from build123d import *

# Parameters (mm, degrees)
BOSS_EXTRUDE1_DEPTH   = 4
BOSS_EXTRUDE1_2_DEPTH = 4
BOSS_EXTRUDE3_DEPTH   = 4
FILLET2_R             = 1
SKETCH4_W             = 14.347682942
SKETCH4_H             = 12.983957321
BOSS_EXTRUDE4_DEPTH   = 15
SKETCH6_W             = 14.347682942
SKETCH6_H             = 3
BOSS_EXTRUDE6_DEPTH   = 10
CUT_EXTRUDE1_REACH    = 49.733
SKETCH7_R             = 1.5
CAVITY2_START         = 21.87499999
CAVITY2_DEPTH         = 1.12500001
SKETCH8_W             = 3
SKETCH8_H             = 13
BOSS_EXTRUDE7_DEPTH   = 10
CUT_EXTRUDE2_REACH    = 71.123
SKETCH10_R            = 1.5


# Read off the part's stored shape, not the designer's step: Cavity2
with BuildPart() as part:
    # Sketch1 → Boss-Extrude1 (new body)
    with BuildSketch(Plane(origin=(0, 0, 0), x_dir=(1, 0, 0), z_dir=(0, 1, 0))):
        with BuildLine():
            Line((-23.6, 10.542278437), (-17, 10.542278437))
            ThreePointArc((-17, 10.542278437), (-15.475, 9.017278437), (-17, 7.492278437))
            Line((-17, 7.492278437), (-23.6, 7.492278437))
            ThreePointArc((-23.6, 7.492278437), (-25.125, 9.017278437), (-23.6, 10.542278437))
        make_face()
    extrude(amount=BOSS_EXTRUDE1_DEPTH)



with BuildPart() as body_2:
    # Sketch1 → Boss-Extrude1 2 (new body)
    with BuildSketch(Plane(origin=(0, 0, 0), x_dir=(1, 0, 0), z_dir=(0, 1, 0))):
        with BuildLine():
            Line((23.6, 7.492278437), (17, 7.492278437))
            ThreePointArc((17, 7.492278437), (15.475, 9.017278437), (17, 10.542278437))
            Line((17, 10.542278437), (23.6, 10.542278437))
            ThreePointArc((23.6, 10.542278437), (25.125, 9.017278437), (23.6, 7.492278437))
        make_face()
    extrude(amount=BOSS_EXTRUDE1_2_DEPTH)


with BuildPart() as part_1:
    add(part.part)

    add(body_2.part)  # Boss-Extrude3 merges body 2
    # Sketch3 → Boss-Extrude3 (add)
    with BuildSketch(Plane(origin=(0, 4, 0), x_dir=(1, 0, 0), z_dir=(0, 1, 0))):
        with BuildLine():
            ThreePointArc((15.475, 9.017278437), (15.921662159, 7.938940596), (17, 7.492278437))
            Line((17, 7.492278437), (23.6, 7.492278437))
            ThreePointArc((23.6, 7.492278437), (24.678337841, 7.938940596), (25.125, 9.017278437))
            Line((25.125, 9.017278437), (25.125, 17.305889592))
            Line((25.125, 17.305889592), (25.125, 34.117278437))
            Line((25.125, 34.117278437), (-25.125, 34.117278437))
            Line((-25.125, 34.117278437), (-25.125, 17.305889592))
            Line((-25.125, 17.305889592), (-25.125, 9.017278437))
            ThreePointArc((-25.125, 9.017278437), (-24.678337841, 10.095616278), (-23.6, 10.542278437))
            Line((-23.6, 10.542278437), (-17, 10.542278437))
            ThreePointArc((-17, 10.542278437), (-15.921662159, 10.095616278), (-15.475, 9.017278437))
            Line((-15.475, 9.017278437), (-15.475, 14.117278437))
            Line((-15.475, 14.117278437), (15.475, 14.117278437))
            Line((15.475, 14.117278437), (15.475, 9.017278437))
        make_face()
        with BuildLine():
            Line((-17, 10.542278437), (-23.6, 10.542278437))
            ThreePointArc((-23.6, 10.542278437), (-25.125, 9.017278437), (-23.6, 7.492278437))
            Line((-23.6, 7.492278437), (-17, 7.492278437))
            ThreePointArc((-17, 7.492278437), (-15.475, 9.017278437), (-17, 10.542278437))
        make_face()
    extrude(amount=BOSS_EXTRUDE3_DEPTH)

    # Fillet2
    fillet2_edges = [part_1.edges().sort_by_distance(p)[0] for p in [
        (-25.125, 8, -21.567278437),
        (15.475, 8, -11.567278437),
        (-24.678337841, 8, -7.938940596),
        (-20.3, 8, -7.492278437),
        (-15.921662159, 8, -7.938940596),
        (-15.475, 8, -11.567278437),
        (15.921662159, 8, -7.938940596),
        (20.3, 8, -7.492278437),
        (24.678337841, 8, -7.938940596),
        (25.125, 8, -21.567278437),
    ]]
    fillet(fillet2_edges, radius=FILLET2_R)

    # Sketch4 → Boss-Extrude4 (add)
    with BuildSketch(Plane(origin=(0, 8, 0), x_dir=(1, 0, 0), z_dir=(0, 1, 0))):
        with Locations((-7.885296824, 27.625299777)):
            Rectangle(SKETCH4_W, SKETCH4_H)
    extrude(amount=BOSS_EXTRUDE4_DEPTH)

    # Sketch6 → Boss-Extrude6 (add)
    with BuildSketch(Plane(origin=(0, 23, 0), x_dir=(1, 0, 0), z_dir=(0, 1, 0))):
        with Locations((-7.885296824, 32.617278437)):
            Rectangle(SKETCH6_W, SKETCH6_H)
    extrude(amount=BOSS_EXTRUDE6_DEPTH)

    # Sketch7 → Cut-Extrude1 (cut, up to next)
    with BuildSketch(Plane.XY.offset(-31.117278437), mode=Mode.PRIVATE) as cut_extrude1_sk1:
        with Locations((-11.819138295, 28.245)):
            Circle(SKETCH7_R)
    cut_extrude1_tool1 = extrude(cut_extrude1_sk1.sketch, amount=-CUT_EXTRUDE1_REACH, mode=Mode.PRIVATE) & part_1.part
    # Sketch7 → Cut-Extrude1 (cut, up to next)
    with BuildSketch(Plane.XY.offset(-31.117278437), mode=Mode.PRIVATE) as cut_extrude1_sk2:
        with Locations((-5.789138295, 28.245)):
            Circle(SKETCH7_R)
    cut_extrude1_tool2 = extrude(cut_extrude1_sk2.sketch, amount=-CUT_EXTRUDE1_REACH, mode=Mode.PRIVATE) & part_1.part
    add(cut_extrude1_tool1.solids().sort_by_distance((-11.819138, 28.245, -31.117278))[0], mode=Mode.SUBTRACT)
    add(cut_extrude1_tool2.solids().sort_by_distance((-5.789138, 28.245, -31.117278))[0], mode=Mode.SUBTRACT)

    # Cavity2 outline → Cavity2 (cut)
    with BuildSketch(Plane(origin=(0, 0, 0), x_dir=(1, 0, 0), z_dir=(0, 1, 0)).offset(CAVITY2_START)):
        Polygon((-0.711455353, 21.133321116), (-0.711455353, 31.117278437), (-14.875000136, 31.117278437), (-14.874999824, 29.504253116), (-14.874998603, 27.254253271), (-14.869868878, 27.115654486), (-14.854507644, 26.977814263), (-14.829001512, 26.841486537), (-14.793485992, 26.707417297), (-14.748156659, 26.57633996), (-14.693263575, 26.448972009), (-14.629105695, 26.326010144), (-14.55603366, 26.208127189), (-14.474448405, 26.095968178), (-14.384794172, 25.99014676), (-14.287564095, 25.89124194), (-14.183289029, 25.799794912), (-14.072538942, 25.716306013), (-13.955921523, 25.641232065), (-13.8340724, 25.574983827), (-4.891452092, 21.133285849), align=None)
    extrude(amount=CAVITY2_DEPTH, mode=Mode.SUBTRACT)

    # Sketch8 → Boss-Extrude7 (add)
    with BuildSketch(Plane.XZ.offset(-4)):
        with Locations((-23.625, -27.617278437)):
            Rectangle(SKETCH8_W, SKETCH8_H)
    extrude(amount=BOSS_EXTRUDE7_DEPTH)

    # Sketch10 → Cut-Extrude2 (cut, up to next)
    with BuildSketch(Plane.ZY.offset(25.125), mode=Mode.PRIVATE) as cut_extrude2_sk1:
        with Locations((-23.44448468, -2.644785648)):
            Circle(SKETCH10_R)
    cut_extrude2_tool1 = extrude(cut_extrude2_sk1.sketch, amount=-CUT_EXTRUDE2_REACH, mode=Mode.PRIVATE) & part_1.part
    # Sketch10 → Cut-Extrude2 (cut, up to next)
    with BuildSketch(Plane.ZY.offset(25.125), mode=Mode.PRIVATE) as cut_extrude2_sk2:
        with Locations((-31.44448468, -2.644785648)):
            Circle(SKETCH10_R)
    cut_extrude2_tool2 = extrude(cut_extrude2_sk2.sketch, amount=-CUT_EXTRUDE2_REACH, mode=Mode.PRIVATE) & part_1.part
    add(cut_extrude2_tool1.solids().sort_by_distance((-25.125, -2.644786, -23.444485))[0], mode=Mode.SUBTRACT)
    add(cut_extrude2_tool2.solids().sort_by_distance((-25.125, -2.644786, -31.444485))[0], mode=Mode.SUBTRACT)


solid = part_1.part
Could you check a few things on this model? Use its own coordinates, in mm. A direction names the side the tool comes from. Give positions to 0.01 mm unless a question says otherwise; leave off trailing zeros. Write each loop counter-clockwise with the first axis right and the second up, starting at its lowest first coordinate (ties: lowest second). Pieces come first, ordered by that corner, then holes. Notation, with made-up numbers: (73.25, -3) -> (117.25, -3) arc R29 cw to (117.25, 32) -> close; hole circle Ø2 at (-17, -36.5). An arc over 180 degrees is marked (long way). Answer as a JSON object with one key per item and string values.
Q1. Suppose I cut it at D-D on z = -16.75. Write out the boundary of the cut face in (x, y) (3 decimals).
Taken from the geometry:
{"outline": "(-25.125, 4) -> (25.125, 4) -> (25.125, 7) arc R1 ccw to (24.125, 8) -> (-24.125, 8) arc R1 ccw to (-25.125, 7) -> close"}
Q2. Will these pins go through, and if not, where does the flat tip stop? pin 1 Ø2.5 at (x, y) = (-23.5, -1.5) entering from +Z; pin 2 Ø4.5 at (x, y) = (-19.5, 2.5) entering from -Z; pin 3 Ø8 at (y, z) = (27, -28) entering from +X; pin 4 Ø1.8 at (y, z) = (-2.64, -23.44) entering from +X.
Taken from the geometry:
{"pin 1": "stops at z = -21.12", "pin 2": "stops at z = -34.12", "pin 3": "stops at x = -0.71", "pin 4": "passes through"}
Q3. Please list where these lines run through material, in increasing order: L1, parallel to Z at x = -7.5, y = 30; L2, parallel to Y at x = 5.5, z = -16.5; L3, parallel to Y at x = -7.5, z = -21.25.
Taken from the geometry:
{"L1": "z = -34.12 to -31.12", "L2": "y = 4 to 8", "L3": "y = 4 to 23"}
Q4. Which directions (+Z, -Z, +X, -X, +Y, -Y) give clear straight access to the entire face, cutting with the end or side of a thin tool? Please do faces 4 (the flat face through (20, 2, -10.542)), 5 (the flat face through (-12, 23, -23)), 6 (the cylindrical face through (-15.58, 2.67, -8.46)).
Taken from the geometry:
{"face 4": "-Z, +X, -X, -Y", "face 5": "+Z, +X, -X, +Y", "face 6": "-Y"}
Q5. We'd pull the mould along Y, two halves only. Please class faces 1 (the cylindrical face through (-23.65, -1.63, -32.55)), 2 (the flat face through (-9.425, 22.43, -23.385)), 3 (the flat face through (20, 0, -9)): released by +Y, released by -Y, zero draft, split by the parting line, or undercut.
Taken from the geometry:
{"face 1": "undercut", "face 2": "zero draft", "face 3": "released by -Y"}
Q6. Suppose I cut it at B-B on x = 19.5. Write out the boundary of the cut face in (y, z).
Taken from the geometry:
{"outline": "(0, -10.54) -> (4, -10.54) -> (4, -34.12) -> (8, -34.12) -> (8, -8.49) arc R1 ccw to (7, -7.49) -> (0, -7.49) -> close"}
Q7. Suppose I cut it at A-A on z = -12. Write out the boundary of the cut face in (x, y) (3 decimals), then the cut area to 3 significant figures.
Taken from the geometry:
{"outline": "(-25.125, 4) -> (-15.475, 4) -> (-15.475, 7) arc R1 ccw to (-16.475, 8) -> (-24.125, 8) arc R1 ccw to (-25.125, 7) -> close; (15.475, 4) -> (25.125, 4) -> (25.125, 7) arc R1 ccw to (24.125, 8) -> (16.475, 8) arc R1 ccw to (15.475, 7) -> close", "area": "76.3 mm²"}
Q8. Suppose I cut it at C-C on x = -12. Write out the boundary of the cut face in (y, z) (3 decimals).
Taken from the geometry:
{"outline": "(4, -34.117) -> (26.756, -34.117) -> (26.756, -31.117) -> (21.875, -31.117) -> (21.875, -24.664) -> (23, -24.664) -> (23, -21.133) -> (8, -21.133) -> (8, -14.117) -> (4, -14.117) -> close; (29.734, -34.117) -> (33, -34.117) -> (33, -31.117) -> (29.734, -31.117) -> close"}
